from build123d import *

# Parameters (mm, degrees)
SKETCH2_R           = 0.25
BOSS_EXTRUDE1_DEPTH = 5


with BuildPart() as part:
    # Sketch1 → Revolve1 (revolve)
    with BuildSketch(Plane(origin=(0, 0, 0), x_dir=(0, 0, -1), z_dir=(1, 0, 0))):
        with BuildLine():
            Line((-2.5, -0.431829007), (-2.5, 5.568170993))
            ThreePointArc((-2.5, 5.568170993), (-1.767766953, 7.335937946), (0, 8.068170993))
            Line((0, 8.068170993), (0, 1.631287774))
            Line((0, 1.631287774), (0, -1.431829007))
            Line((0, -1.431829007), (-2.65, -1.431829007))
            Line((-2.65, -1.431829007), (-2.65, -0.431829007))
            Line((-2.65, -0.431829007), (-2.5, -0.431829007))
        make_face()
    revolve(axis=Axis((0, 8.068170993, 0), (0, -1, 0)))

    # Sketch2 → Boss-Extrude1 (add)
    with BuildSketch(Plane.XZ.offset(1.431829007)):
        with Locations(Location((-1.5, 0, 0), (0, 0, 270))):
            Circle(SKETCH2_R)
        with Locations(Location((1.5, 0, 0), (0, 0, 90))):
            Circle(SKETCH2_R)
    extrude(amount=BOSS_EXTRUDE1_DEPTH)


solid = part.part
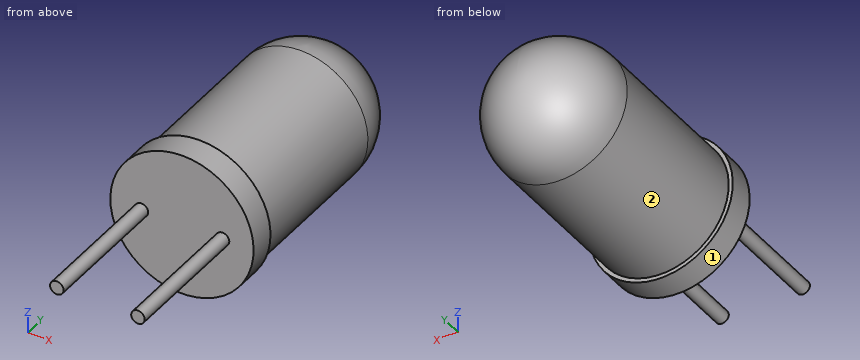
Input: part model. Units: mm. Frame: model coordinates. Face numbers are marked on the shaded views. A direction names the side the tool comes from. Give positions to 0.01 mm unless a question says otherwise; leave off trailing zeros. Loops run counter-clockwise (first coordinate to the right, second up) from the corner with the lowest first, then second, coordinate; pieces in that order, holes last. Notation, with made-up numbers: (-24, 23.25) -> (-11, 23.25) arc R36 cw to (-11, 59.25) -> close; hole circle Ø7 at (43, 3.25). An arc over 180 degrees is marked (long way). Answer as a JSON object with one key per item and string values. Group by question number.
Item 1: Pin query (flat end, axial travel): P1, Ø1.6, axis at x = -0.5, z = -1, coming from the +Y side; P2, Ø3, axis at x = 2, y = -2, coming from the -Z side; P3, Ø1.5, axis at x = -1, y = -4, coming from the +Z side. Return the tip coordinate at first contact, or that it passes through.
Item 2: Cut plane D-D, the plane y = 1.25. Return the cut outline in (x, z).
Item 3: Line query: probe 1 along Y at (x, z) = (2.3, -1.05); probe 2 along Z at (x, y) = (1.6, -2.5); probe 3 along Z at (x, y) = (-1.7, 2.5). Output: solid intervals per line, ascending.
Item 4: Cut plane A-A, the plane z = 0. Return the cut outline in (x, y).
Item 5: Reachability of the marked faces 1 and 2 from +Z, -Z, +X, -X, +Y, -Y: full face, straight path, thin tool, end or side. Return the list, or none.
Item 6: Cut plane B-B, the plane x = 0. Return the cut outline in (y, z).
Item 7: Cut plane C-C, the plane y = -2. Return the cut outline in (x, z).
Checks:
{
 "1": {"P1": "stops at y = 8.05", "P2": "stops at z = -2.58", "P3": "stops at z = 0.25"},
 "2": {"outline": "circle Ø5 at (0, 0)"},
 "3": {"probe 1": "y = -1.43 to -0.43", "probe 2": "z = -0.23 to 0.23", "probe 3": "z = -1.83 to 1.83"},
 "4": {"outline": "(-2.65, -1.43) -> (-1.75, -1.43) -> (-1.75, -6.43) -> (-1.25, -6.43) -> (-1.25, -1.43) -> (1.25, -1.43) -> (1.25, -6.43) -> (1.75, -6.43) -> (1.75, -1.43) -> (2.65, -1.43) -> (2.65, -0.43) -> (2.5, -0.43) -> (2.5, 5.57) arc R2.5 ccw to (-2.5, 5.57) -> (-2.5, -0.43) -> (-2.65, -0.43) -> close"},
 "5": {"face 1": "+Y, -Y", "face 2": "+Y"},
 "6": {"outline": "(-1.43, -2.65) -> (-0.43, -2.65) -> (-0.43, -2.5) -> (5.57, -2.5) arc R2.5 ccw to (5.57, 2.5) -> (-0.43, 2.5) -> (-0.43, 2.65) -> (-1.43, 2.65) -> close"},
 "7": {"outline": "circle Ø0.5 at (-1.5, 0); circle Ø0.5 at (1.5, 0)"}
}
